```python
from build123d import *

# Parameters (mm, degrees)
F0_R     = 0.649287
F1_DEPTH = 3.81
F0_R_2   = 6.031813
F2_DEPTH = 2.54
F0_R_3   = 9.525
F3_DEPTH = 3.81
F4_R     = 0.254


with BuildPart() as f1:
    # F0 (on Right) → F1 (new body, symmetric)
    with BuildSketch(Plane.YZ):
        Circle(F0_R)
    extrude(amount=F1_DEPTH, both=True)

    # F0 (on Right) → F2 (join, symmetric)
    with BuildSketch(Plane.YZ):
        Circle(F0_R_2)
        Circle(F0_R, mode=Mode.SUBTRACT)
    extrude(amount=F2_DEPTH, both=True)

    # F0 (on Right) → F3 (join, symmetric)
    with BuildSketch(Plane.YZ):
        Circle(F0_R_3)
        Circle(F0_R_2, mode=Mode.SUBTRACT)
    extrude(amount=F3_DEPTH, both=True)

    # F4
    f4_edges = [f1.edges().sort_by_distance(p)[0] for p in [
        (3.81, -9.525, 0),
        (-3.81, -9.525, 0),
    ]]
    fillet(f4_edges, radius=F4_R)


solid = f1.part
```
Here's how the part is built. I have some questions about the finished solid (model axes, mm). A direction names the side the tool comes from. Coordinates: 2 decimals unless noted, no trailing zeros. Order: outer loops, then holes, each group sorted by start corner. A loop starts at its lowest first (then second) coordinate and runs counter-clockwise, first axis right, second up. Notation, with made-up numbers: (3.25, 86.5) - (23.25, 86.5) arc R8 ccw to (23.25, 98.5) - close; hole circle Ø2 at (68, 19.25). An arc over 180 degrees is marked (long way). One line per question, with ' | ' between items. Start each with the question number.
1. Which directions (+Z, -Z, +X, -X, +Y, -Y) give clear straight access to the entire face, cutting with the end or side of a thin tool? Please do faces 1 (the flat face through (3.81, 2, -6)), 2 (the cylindrical face through (3.17, -0.79, 5.98)), 3 (the flat face through (-2.54, 1, 0)).
2. If we section it at C-C (x = -1.5): Write out the boundary of the cut face in (y, z) (3 decimals), and give its area (3 significant figures).
3. If we section it at A-A (y = 0): Write out the boundary of the cut face in (x, z) (3 decimals), and give its area (3 significant figures).
4. I'm going to push flat-ended pins straight in: pin 1 Ø4 at (y, z) = (1.5, -2.5) entering from +X; pin 2 Ø9.5 at (y, z) = (0, -2) entering from -X; pin 3 Ø1 at (x, z) = (2, 5.5) entering from +Y; pin 4 Ø1 at (x, y) = (-1.5, -6.5) entering from -Z. Where does each tip first touch, or does it pass through?
5. Please list where these lines run through material, in increasing order: line 1 along Z through (x, y) = (3.55, 0) (3 decimals); line 2 along X through (y, z) = (0.5, 2); line 3 along Y through (x, z) = (3.75, 4.75). Write a range as [from, to].
6. If we mould it in two halves opening along Z, with no side actions, what happens to faces 4 (the flat face through (3.81, 0, 0)), 5 (the cylindrical face through (-3.166, -0.515, -0.395)), 6 (the cylindrical face through (0.05, -7.559, -5.796))? For each: released by +Z, released by -Z, zero draft, split by the parting line, or undercut.
Model answer:
1) face 1: +Z, -Z, +X, +Y, -Y | face 2: +X | face 3: -X
2) outline: circle Ø19.05 at (0, 0) | area: 285 mm²
3) outline: (-3.81, -9.271) arc R0.254 ccw to (-3.556, -9.525) - (3.556, -9.525) arc R0.254 ccw to (3.81, -9.271) - (3.81, -6.032) - (2.54, -6.032) - (2.54, -0.649) - (3.81, -0.649) - (3.81, 0.649) - (2.54, 0.649) - (2.54, 6.032) - (3.81, 6.032) - (3.81, 9.271) arc R0.254 ccw to (3.556, 9.525) - (-3.556, 9.525) arc R0.254 ccw to (-3.81, 9.271) - (-3.81, 6.032) - (-2.54, 6.032) - (-2.54, 0.649) - (-3.81, 0.649) - (-3.81, -0.649) - (-2.54, -0.649) - (-2.54, -6.032) - (-3.81, -6.032) - close | area: 118 mm²
4) pin 1: stops at x = 2.54 | pin 2: stops at x = -3.81 | pin 3: stops at y = 8.11 | pin 4: stops at z = -7.4
5) line 1: z = [-9.525, -6.032], [-0.649, 0.649], [6.032, 9.525] | line 2: x = [-2.54, 2.54] | line 3: y = [-8.15, -3.72], [3.72, 8.15]
6) face 4: zero draft | face 5: undercut | face 6: split by the parting line
